Part model, mm, in its own coordinate system. A direction names the side the tool comes from. Give positions to 0.01 mm unless a question says otherwise; leave off trailing zeros. Order: outer loops, then holes, each group sorted by start corner. A loop starts at its lowest first (then second) coordinate and runs counter-clockwise, first axis right, second up. Notation, with made-up numbers: (17.5, 1.25) - (63.5, 1.25) arc R18 cw to (63.5, 24.25) - close; hole circle Ø5 at (60.5, 70). An arc over 180 degrees is marked (long way). Use one line per item in the form item = value. Start each with the question number.
1. Band-saw the part on D-D, the plane z = 5. State how many separate pieces and enclosed holes the cut face has, plus the area to 3 significant figures.
2. Tool access for faces 1 (the face through (0, 2, 3)), 2 (the face through (0, 3.25, 1)), 3 (the face through (21, 0, 1)), 4 (the face through (-0.29, 3.25, 5.75)): list every direction of +Z, -Z, +X, -X, +Y, -Y with a clear straight run to the whole face (end or side of a thin tool).
3. Pull direction Y, two halves, no side cores. Call faces 5 (the face through (21.474, -0.481, 1.014)), 6 (the face through (0, 2, 6)), 7 (the face through (0.29, -3.25, 5.75)): +Y half, -Y half, draft (parallel to the pull), parting line (faces both ways), or undercut.
4. Band-saw the part on B-B, the plane y = 0. List the corners of the cut face in (x, z), plus the area to 3 significant figures.
5. Band-saw the part on A-A, the plane x = 0. List the corners of the cut face in (y, z).
6. Drill centre lines: line 1 (Y direction, x = -8.5, z = 3.5); line 2 (Y direction, x = -8, z = 1.75); line 3 (X direction, y = 0.25, z = 1.75). Where is each one in solid material? Low to high.
7. Pin check, flat tips, straight feed: P1, Ø6, axis at x = -8, y = -4, coming from the +Z side; P2, Ø2, axis at x = 0, y = 2, coming from the -Z side; P3, Ø3, axis at x = -23, y = 0, coming from the +Z side; P4, Ø2.5, axis at x = 0, z = 4.5, coming from the -Y side. Stop position of each tip, or through.
8. Band-saw the part on C-C, the plane x = 23. List the corners of the cut face in (y, z).
Autodesk Inventor part; units mm, degrees
ref_plane "YZ Plane" through (0, 0, 0) normal (1, 0, 0) x (0, 1, 0)
ref_plane "XZ Plane" through (0, 0, 0) normal (0, 1, 0) x (-1, 0, 0)
ref_plane "XY Plane" through (0, 0, 0) normal (0, 0, 1) x (1, 0, 0)
sketch "Эскиз1" plane through (0, 0, 0) normal (0, 0, 1) x (1, 0, 0)
  line L0 (-30, -12.5) -> (30, -12.5) construction
  line L1 (30, -12.5) -> (30, 12.5) construction
  line L2 (30, 12.5) -> (-30, 12.5) construction
  line L3 (-30, 12.5) -> (-30, -12.5) construction
  line L4 (-30, -12.5) -> (30, 12.5) construction
  line L5 (30, -12.5) -> (-30, 12.5) construction
  line L6 (-25, 5.25) -> (25, 5.25)
  line L7 (25, 5.25) -> (25, -5.25)
  line L8 (25, -5.25) -> (-25, -5.25)
  line L9 (-25, -5.25) -> (-25, 5.25)
  line L10 (-25, 5.25) -> (25, -5.25) construction
  line L11 (25, 5.25) -> (-25, -5.25) construction
  line L12 (21, 3.25) -> (-21, 3.25)
  line L13 (-21, -3.25) -> (21, -3.25)
  line L14 (21, 3.25) -> (21, -3.25)
  line L15 (-21, 3.25) -> (-21, -3.25)
  point P0 (0, 0)
  dimension "d0" = 60
  dimension "d1" = 25
  dimension "d2" = 50
  dimension "d3" = 10.5
  dimension "d4" = 2
  dimension "d15" = 4
  dimension "d16" = 4
  dimension "d27" = 2
extrude "Выдавливание1" add sketch "Эскиз1" along normal blind 2
sketch "Эскиз4" plane through (0, 0, 2) normal (0, 0, 1) x (1, 0, 0)
  circle A0 centre (-23, 0) radius 1.6
  line L0 (-21, -3.25) -> (-21, 3.25)
  point P0 (0, 0)
  dimension "d17" = 3.2
  dimension "d18" = 2
extrude "Выдавливание3" cut sketch "Эскиз4" against normal blind 3
mirror "Зеркальное отражение2" about plane through (0, 0, 0) normal (1, 0, 0) of "Выдавливание3"
chamfer "Фаска2" distance 0.5 angle 45 4 edges at (25, -5.25, 1) (-25, -5.25, 1) (-25, 5.25, 1) (25, 5.25, 1)
sketch "Эскиз2" plane through (-25, 5.25, 0) normal (0, 1, 0) x (1, 0, 0)
  spline S0 degree 4 poles (46, 0) (42.3251, -1.5041) (33.5066, -3.3836) (31.2881, -3) (28, -3) knots 0 0 0 0 0 1 1 1 1 1
  line L0 (25, 0) -> (25, -3) construction
  line L1 (25, -3) -> (28, -3)
  line L2 (26.5, -6) -> (23.5, -6)
  line L3 (25, -3) -> (25, -6)
  spline S1 degree 4 poles (26.5, -6) (32.4688, -6) (38.7503, -3.3818) (43.4963, -3.2883) (46, -2) knots 0 0 0 0 0 1 1 1 1 1
  circle A0 centre (25, -4.5) radius 1.1
  line L4 (46, 0) -> (46, -2)
  line L5 (50, -2) -> (0, -2)
  spline S2 degree 4 poles (4, 0) (7.6749, -1.5041) (16.4934, -3.3836) (18.7119, -3) (22, -3) knots 0 0 0 0 0 1 1 1 1 1
  line L6 (25, -3) -> (22, -3)
  line L7 (23.5, -6) -> (26.5, -6)
  spline S3 degree 4 poles (23.5, -6) (17.5312, -6) (11.2497, -3.3818) (6.5037, -3.2883) (4, -2) knots 0 0 0 0 0 1 1 1 1 1
  line L8 (4, 0) -> (4, -2)
  line L9 (50, 0) -> (0, 0)
  point P0 (37.5638, -2.2507)
  point P1 (31.2637, -3)
  point P2 (36.2453, -4.5)
  point P3 (42.8648, -3)
  point P4 (26.5, -3)
  point P5 (38.8382, -2)
  point P6 (12.4362, -2.2507)
  point P7 (18.7363, -3)
  point P8 (13.7547, -4.5)
  point P9 (7.1352, -3)
  point P10 (11.1618, -2)
  point P11 (4, -2)
  point P12 (23.5, -9)
  point P13 (4, -2)
  point P14 (45.3365, 0)
  point P15 (4, 0)
  point P16 (23.5, -3)
  point P17 (26.5, -6)
  dimension "d7" = 3
  dimension "d8" = 2.2
  dimension "d9" = 3
  dimension "d10" = 3
  dimension "d32" = 2
  dimension "d39" = 1
extrude "Выдавливание7" add sketch "Эскиз2" against normal blind 4 contours L4 L5 S0 | L5 S1 L2 L3 A0 L1 S0 | S2 L5 L8 | S2 L6 L3 A0 L2 S3 L5
extrude "Выдавливание8" cut sketch "Эскиз2" against normal blind 2 contours L5 S1 L2 L3 A0 L1 S0 | S2 L6 L3 A0 L2 S3 L5
mirror "Зеркальное отражение5" about plane through (0, 0, 0) normal (0, 1, 0) of "Выдавливание7", "Выдавливание8"
properties part number "мост"
From the geometry:
q1.separate_pieces = 4
q1.enclosed_holes = 0
q1.area = 63.9 mm²
q2.face_1 = -Z, +Y, -Y
q2.face_2 = -Z
q2.face_3 = +Z, -Z
q2.face_4 = +Z, +X, -X, +Y
q3.face_5 = undercut
q3.face_6 = draft
q3.face_7 = -Y half
q4.outline = (-25, 0) - (-24.6, 0) - (-24.6, 2) - (-25, 2) - close; (-21.4, 0) - (-21, 0) - (-21, 2) - (-21.4, 2) - close; (21, 0) - (21.4, 0) - (21.4, 2) - (21, 2) - close; (24.6, 0) - (25, 0) - (25, 2) - (24.6, 2) - close
q4.area = 3.20 mm²
q5.outline = (-5.25, 0) - (-3.25, 0) - (-3.25, 2) - (-5.25, 2) - close; (-3.25, 3) - (-1.25, 3) - (-1.25, 3.4) - (-3.25, 3.4) - close; (-3.25, 5.6) - (-1.25, 5.6) - (-1.25, 6) - (-3.25, 6) - close; (1.25, 3) - (3.25, 3) - (3.25, 3.4) - (1.25, 3.4) - close; (1.25, 5.6) - (3.25, 5.6) - (3.25, 6) - (1.25, 6) - close; (3.25, 0) - (5.25, 0) - (5.25, 2) - (3.25, 2) - close
q6.line_1 = -3.25 to -1.25, 1.25 to 3.25
q6.line_2 = -5.25 to -3.25, 3.25 to 5.25
q6.line_3 = -25 to -24.58, -21.42 to -21, 21 to 21.42, 24.58 to 25
q7.P1 = 5.71
q7.P2 = 3
q7.P3 = through
q7.P4 = -3.25
q8.outline = (-5.25, 0) - (-1.6, 0) - (-1.6, 2) - (-5.25, 2) - close; (1.6, 0) - (5.25, 0) - (5.25, 2) - (1.6, 2) - close
